Geometry: final body of the model. Coordinates: model frame, mm. A direction names the side the tool comes from. Coordinates: 2 decimals unless noted, no trailing zeros. Order: outer loops, then holes, each group sorted by start corner. A loop starts at its lowest first (then second) coordinate and runs counter-clockwise, first axis right, second up. Notation, with made-up numbers: (-14.75, 8.25) -> (5.25, 8.25) arc R12 cw to (5.25, 13.25) -> close; hole circle Ø6 at (28.5, 0.25). An arc over 180 degrees is marked (long way). Use one line per item in the form item = value.
```python
from build123d import *

# Parameters (mm, degrees)
SKETCH1_W           = 15.85
SKETCH1_H           = 7.85
BOSS_EXTRUDE1_DEPTH = 3.15
SHELL1_T            = -1.5
SKETCH2_R           = 2.45
SKETCH2_R_2         = 1.55
BOSS_EXTRUDE2_DEPTH = 1.8


with BuildPart() as part:
    # Sketch1 → Boss-Extrude1 (new body)
    with BuildSketch(Plane(origin=(0, 0, 0), x_dir=(1, 0, 0), z_dir=(0, 1, 0))):
        Rectangle(SKETCH1_W, SKETCH1_H)
    extrude(amount=-BOSS_EXTRUDE1_DEPTH)

    # Shell1
    shell1_openings = [part.faces().sort_by_distance(p)[0] for p in [
        (0, -3.15, 0),
    ]]
    offset(amount=SHELL1_T, openings=shell1_openings, kind=Kind.INTERSECTION)

    # Sketch2 → Boss-Extrude2 (add)
    with BuildSketch(Plane(origin=(0, 0, 0), x_dir=(1, 0, 0), z_dir=(0, 1, 0))):
        with Locations(Location((0, 0, 0), (0, 0, 270))):
            Circle(SKETCH2_R)
        with Locations(Location((0, 0, 0), (0, 0, 270))):
            Circle(SKETCH2_R_2, mode=Mode.SUBTRACT)
    extrude(amount=BOSS_EXTRUDE2_DEPTH)


solid = part.part
```
1) Section B-B, the plane x = 3.25. Output: boundary loops of the cut face in (y, z) (3 decimals).
Results found:
outline = (-3.15, -3.925) -> (0, -3.925) -> (0, 3.925) -> (-3.15, 3.925) -> (-3.15, 2.425) -> (-1.5, 2.425) -> (-1.5, -2.425) -> (-3.15, -2.425) -> close
2) Contact query for flat-ended pins moving along their axis: P1, Ø3.5, axis at x = -0.5, z = 0.5, coming from the +Y side; P2, Ø2.5, axis at x = -0.5, z = 0.5, coming from the -Y side; P3, Ø1.5, axis at y = 1, z = 2.5, coming from the -X side. Output: stop coordinate, or through.
Results found:
P1 = 1.8
P2 = -1.5
P3 = -1.71
3) Pull-direction query (Z, two-part tool) for faces 1 (the cylindrical face through (0.736, 0.887, 2.337)), 2 (the flat face through (0, -2, 2.425)), 3 (the flat face through (-2, 1.8, 0)); classes: released by +Z, released by -Z, zero draft, split by the parting line, or undercut.
Results found:
face_1 = split by the parting line
face_2 = undercut
face_3 = zero draft
4) Section C-C, the plane z = 0. Output: boundary loops of the cut face in (x, y) (3 decimals).
Results found:
outline = (-7.925, -3.15) -> (-6.425, -3.15) -> (-6.425, -1.5) -> (6.425, -1.5) -> (6.425, -3.15) -> (7.925, -3.15) -> (7.925, 0) -> (2.45, 0) -> (2.45, 1.8) -> (1.55, 1.8) -> (1.55, 0) -> (-1.55, 0) -> (-1.55, 1.8) -> (-2.45, 1.8) -> (-2.45, 0) -> (-7.925, 0) -> close
5) Section A-A, the plane y = -1.75. Output: boundary loops of the cut face in (x, z) (3 decimals), and give its area (3 significant figures).
Results found:
outline = (-7.925, -3.925) -> (7.925, -3.925) -> (7.925, 3.925) -> (-7.925, 3.925) -> close; hole (-6.425, -2.425) -> (6.425, -2.425) -> (6.425, 2.425) -> (-6.425, 2.425) -> close
area = 62.1 mm2
6) Access query for faces 4 (the flat face through (6.425, -2, 0)), 5 (the flat face through (-7.925, -2, 0)), 6 (the flat face through (0, 0, 0)). Directions: +Z, -Z, +X, -X, +Y, -Y. A direction counts if a zero-diameter tool reaches every point of the face in a straight line with its end or side. Return the directions, or none.
Results found:
face_4 = -Y
face_5 = +Z, -Z, -X, +Y, -Y
face_6 = +Y
7) Material intervals for probe 1 along X at (y, z) = (1.1, 0); probe 2 along Z at (x, y) = (3.25, -1.65) (3 decimals); probe 3 along Y at (x, z) = (-5.25, -3.25), sorted ascending. Write a range as from..to.
Results found:
probe_1 = -2.45..-1.55, 1.55..2.45
probe_2 = -3.925..-2.425, 2.425..3.925
probe_3 = -3.15..0
8) Section D-D, the plane x = 0. Output: boundary loops of the cut face in (y, z) (3 decimals).
Results found:
outline = (-3.15, -3.925) -> (0, -3.925) -> (0, -2.45) -> (1.8, -2.45) -> (1.8, -1.55) -> (0, -1.55) -> (0, 1.55) -> (1.8, 1.55) -> (1.8, 2.45) -> (0, 2.45) -> (0, 3.925) -> (-3.15, 3.925) -> (-3.15, 2.425) -> (-1.5, 2.425) -> (-1.5, -2.425) -> (-3.15, -2.425) -> close
